```python
from build123d import *

# Parameters (mm, degrees)
EXTRUDE_1_DEPTH          = 6
CUT_EXTRUDE_1_DEPTH      = 4
SKETCH_3_R               = 1.5
CUT_EXTRUDE_2_DEPTH      = 4
SKETCH_5_W               = 9
SKETCH_5_H               = 12
EXTRUDE_2_DEPTH          = 12
CUT_EXTRUDE_3_DEPTH      = 30.816103032
SKETCH_9_R               = 2.5
CUT_EXTRUDE_6_DEPTH      = 24.579652245
CUT_EXTRUDE_7_DEPTH      = 26.475478406
CUT_EXTRUDE_7_DEPTH_BACK = 26.475478406
SKETCH_10_R              = 1.5


with BuildPart() as part:
    # 草图1 → 凸台-拉伸1 (new body)
    with BuildSketch(Plane(origin=(0, 0, 0), x_dir=(1, 0, 0), z_dir=(0, 1, 0))):
        with BuildLine():
            ThreePointArc((0, -6), (-6, 0), (0, 6))
            Line((0, 6), (-6, 6))
            Line((-6, 6), (-17, 6))
            Line((-17, 6), (-17, -6))
            Line((-17, -6), (0, -6))
        make_face()
        with BuildLine():
            Line((0, -6), (0, 0))
            Line((0, 0), (0, 6))
            ThreePointArc((0, 6), (-6, 0), (0, -6))
        make_face()
        with BuildLine():
            Line((0, 6), (0, 0))
            Line((0, 0), (0, -6))
            ThreePointArc((0, -6), (4.242640687, -4.242640687), (6, 0))
            ThreePointArc((6, 0), (4.242640687, 4.242640687), (0, 6))
        make_face()
    extrude(amount=EXTRUDE_1_DEPTH)

    # 草图2 → 切除-拉伸1 (cut)
    with BuildSketch(Plane(origin=(0, 6, 0), x_dir=(1, 0, 0), z_dir=(0, 1, 0))):
        Polygon((2.5, -4.330127019), (5, 0), (2.5, 4.330127019), (-2.5, 4.330127019), (-5, 0), (-2.5, -4.330127019), align=None)
    extrude(amount=-CUT_EXTRUDE_1_DEPTH, mode=Mode.SUBTRACT)

    # 草图3 → 切除-拉伸2 (cut)
    with BuildSketch(Plane.XZ):
        with Locations(Location((0, 0, 0), (0, 0, 270))):
            Circle(SKETCH_3_R)
    extrude(amount=-CUT_EXTRUDE_2_DEPTH, mode=Mode.SUBTRACT)

    # 草图5 → 凸台-拉伸2 (add)
    with BuildSketch(Plane(origin=(0, 6, 0), x_dir=(1, 0, 0), z_dir=(0, 1, 0))):
        with Locations((-12.5, 0)):
            Rectangle(SKETCH_5_W, SKETCH_5_H)
    extrude(amount=EXTRUDE_2_DEPTH)

    # 草图6 → 切除-拉伸3 (cut, through all)
    with BuildSketch(Plane.ZY.offset(17)):
        with BuildLine():
            Line((0, 18), (-6, 18))
            Line((-6, 18), (-6, 12))
            ThreePointArc((-6, 12), (-4.242640687, 16.242640687), (0, 18))
        make_face()
        with BuildLine():
            Line((6, 18), (0, 18))
            ThreePointArc((0, 18), (4.242640687, 16.242640687), (6, 12))
            Line((6, 12), (6, 18))
        make_face()
    extrude(amount=-CUT_EXTRUDE_3_DEPTH, mode=Mode.SUBTRACT)

    # 草图9 → 切除-拉伸6 (cut, through all)
    with BuildSketch(Plane(origin=(-8, 0, 0), x_dir=(0, 0, -1), z_dir=(1, 0, 0))):
        with Locations((0, 12)):
            Circle(SKETCH_9_R)
    extrude(amount=-CUT_EXTRUDE_6_DEPTH, mode=Mode.SUBTRACT)

    # 草图10 → 切除-拉伸7 (cut, two sides: drawn at the far end of the back side and taken through both)
    with BuildSketch(Plane.XY.offset(-CUT_EXTRUDE_7_DEPTH_BACK)):
        with Locations((-12.5, 12)):
            Circle(SKETCH_10_R)
    extrude(amount=CUT_EXTRUDE_7_DEPTH + CUT_EXTRUDE_7_DEPTH_BACK, mode=Mode.SUBTRACT)


solid = part.part
```
Design review of the part built by this model. Coordinates are the model's own, in mm. A direction names the side the tool comes from. Round coordinates to 2 decimals unless told otherwise and drop trailing zeros. Write each loop counter-clockwise with the first axis right and the second up, starting at its lowest first coordinate (ties: lowest second). Pieces come first, ordered by that corner, then holes.
Item 1: We need section C-C on x = -12.5. Write out the cut boundary in (y, z), and give its area (3 significant figures).
Item 2: We need section D-D on z = -5. Write out the cut boundary in (x, y).
Item 3: For faces 1 (the cylindrical face through (-12.44, 13.69, 1.84)), 2 (the flat face through (3.73, 4.03, 2.2)), 3 (the flat face through (-4, 6, -3)), list the 3-axis set-ups (+Z, -Z, +X, -X, +Y, -Y) from which the entire face can be reached by the end or side of a thin tool; tool diameter is ignored.
Item 4: The part is to be moulded in two halves that separate along X. For faces 4 (the flat face through (-3.73, 4.03, -2.2)), 5 (the flat face through (-11, 5, 6)), 6 (the flat face through (-8, 9, 0)), 7 (the flat face through (-17, 9, 0)), say which applies: +X half, -X half, draft (parallel to the pull), parting line (faces both ways), or undercut.
Item 5: We need section B-B on z = -0.75. Write out the cut boundary in (x, y), and give its area (3 significant figures).
Item 6: We need section A-A on y = 3.75. Write out the cut boundary in (x, z), and give its area (3 significant figures).
Item 7: For probe 1 along X at (y, z) = (1.45, 0); probe 2 along X at (y, z) = (12, -5); probe 3 along Y at (x, z) = (-2.75, 4), list the stretches that pass through material, from the lowest coordinate up.
Item 8: Clearance check with flat-ended pins moving along their axes: pin 1 Ø4.5 at (x, z) = (-2, 2) entering from +Y; pin 2 Ø6.5 at (y, z) = (12, 0) entering from +X; pin 3 Ø1.8 at (x, z) = (0, 0) entering from -Y. State where each tip first meets the part, or that it passes through.
Returned:
1. outline: (0, -6) - (10.5, -6) - (10.5, -2) arc R2.5 cw to (10.5, 2) - (10.5, 6) - (0, 6) - close; (13.5, -5.81) arc R6 ccw to (13.5, 5.81) - (13.5, 2) arc R2.5 cw to (13.5, -2) - close
1. area: 159 mm2
2. outline: (-17, 0) - (3.32, 0) - (3.32, 6) - (-8, 6) - (-8, 15.32) - (-17, 15.32) - close; hole circle Ø3 at (-12.5, 12)
3. face 1: +X, -X
3. face 2: +Y
3. face 3: +Z, -Z, +X, +Y
4. face 4: undercut
4. face 5: draft
4. face 6: +X half
4. face 7: -X half
5. outline: (-17, 0) - (-1.3, 0) - (-1.3, 2) - (-4.57, 2) - (-4.57, 6) - (-8, 6) - (-8, 9.62) - (-17, 9.62) - close; (-17, 14.38) - (-8, 14.38) - (-8, 17.95) - (-17, 17.95) - close; (1.3, 0) - (5.95, 0) - (5.95, 6) - (4.57, 6) - (4.57, 2) - (1.3, 2) - close
5. area: 161 mm2
6. outline: (-17, -6) - (0, -6) arc R6 ccw to (0, 6) - (-17, 6) - close; hole (-5, 0) - (-2.5, -4.33) - (2.5, -4.33) - (5, 0) - (2.5, 4.33) - (-2.5, 4.33) - close
6. area: 196 mm2
7. probe 1: x = -17 to -1.5, 1.5 to 6
7. probe 2: x = -17 to -14, -11 to -8
7. probe 3: y = 0 to 6
8. pin 1: stops at y = 6
8. pin 2: stops at x = -8
8. pin 3: passes through
